Here's how the part is built. I have some questions about the finished solid (model axes, mm). A direction names the side the tool comes from. Round coordinates to 2 decimals unless told otherwise and drop trailing zeros. Order: outer loops, then holes, each group sorted by start corner. A loop starts at its lowest first (then second) coordinate and runs counter-clockwise, first axis right, second up. Notation, with made-up numbers: M 30,31.25 L 62,31.25 A20 cw 62,42.25 Z; hole C 63.5,32.25 d1. An arc over 180 degrees is marked long. Write item = value, one per line. Start each with the question number.
Item 1: For faces 4 (the face through (-0.43, 61.27, 6.06)), 5 (the face through (-13, 10, -21)), 6 (the face through (13.3, 0.1, 21.8)), which set-ups out of +Z, -Z, +X, -X, +Y, -Y let a thin tool reach every point of the face, with its end or its side?
Item 2: I want a section at D-D, the plane x = 0. State how many separate pieces and enclosed holes the cut face has, plus the area to 3 significant figures.
Item 3: We'd pull the mould along Z, two halves only. Please class faces 1 (the face through (-13, 0, 26)), 2 (the face through (-0.254, 31.933, -3.916)), 3 (the face through (0.228, 49.266, -1.292)): pulls with the +Z half, pulls with the -Z half, needs draft (parallel to the pull), parting line crosses it, or undercut.
Item 4: I'm going to push flat-ended pins straight in: P1, Ø3, axis at x = -9, y = 24.5, coming from the +Z side; P2, Ø5, axis at y = 0, z = -19, coming from the +X side; P3, Ø1.8, axis at x = 13.5, z = 20.5, coming from the +Y side; P4, Ø10, axis at x = -3, z = 2, coming from the -Y side. Where does each tip first touch, or does it pass through?
Item 5: Please list where these lines run through material, in increasing order: L1, parallel to Y at x = 0, z = -7.25; L2, parallel to Y at x = 9, z = 0; L3, parallel to Y at x = -3, z = -1.5.
Item 6: I want a section at A-A, the plane x = -9. List the corners of the cut face in (y, z) for me.
Item 7: I want a section at B-B, the plane y = 58. List the corners of the cut face in (x, z) for me.
Item 8: I want a section at C-C, the plane z = 19. List the corners of the cut face in (x, y) for me.
```python
from build123d import *

# Parameters (mm, degrees)
EXTRUDE1_DEPTH      = 10.3
EXTRUDE1_DEPTH_BACK = 10.3
SKETCH1_W           = 20
SKETCH1_H           = 55
EXTRUDE2_DEPTH      = 6
SKETCH4_R           = 2.8
EXTRUDE3_DEPTH      = 78.478061411
SKETCH5_R           = 5
EXTRUDE4_DEPTH      = 77.326797391
FILLET2_R           = 1.5
CHAMFER1_SIZE       = 2
SKETCH7_R           = 1.95
EXTRUDE5_DEPTH      = 77.326797413
SKETCH8_R           = 3.3
EXTRUDE6_DEPTH      = 8


with BuildPart() as part:
    # Sketch1 → Extrude1 (new, two sides: drawn at the far end of the back side and taken through both)
    with BuildSketch(Plane(origin=(0, 0, 0), x_dir=(0, 0, -1), z_dir=(1, 0, 0)).offset(-EXTRUDE1_DEPTH_BACK)):
        with Locations((0, 37.8)):
            Rectangle(SKETCH1_W, SKETCH1_H)
    extrude(amount=EXTRUDE1_DEPTH + EXTRUDE1_DEPTH_BACK)

    # Sketch2 → Extrude2 (add)
    with BuildSketch(Plane(origin=(10.3, 0, 0), x_dir=(0, 0, -1), z_dir=(1, 0, 0))):
        with BuildLine():
            Line((26, 10), (17, 10))
            ThreePointArc((17, 10), (12.050252532, 12.050252532), (10, 17))
            Line((10, 17), (10, 65.3))
            Line((10, 65.3), (-10, 65.3))
            Line((-10, 65.3), (-10, 17))
            ThreePointArc((-10, 17), (-12.050252532, 12.050252532), (-17, 10))
            Line((-17, 10), (-26, 10))
            Line((-26, 10), (-26, -10))
            Line((-26, -10), (26, -10))
            Line((26, -10), (26, 10))
        make_face()
    extrude2 = extrude(amount=EXTRUDE2_DEPTH)

    # Mirror2: Extrude2 across plane
    add(extrude2.mirror(Plane(origin=(0, 0, 0), x_dir=(0, 0, 1), z_dir=(1, 0, 0))))

    # Sketch4 → Extrude3 (cut, through all)
    with BuildSketch(Plane(origin=(16.3, 0, 0), x_dir=(0, 0, -1), z_dir=(1, 0, 0))):
        Circle(SKETCH4_R)
        with Locations((19, 0)):
            Circle(SKETCH4_R)
        with Locations((-19, 0)):
            Circle(SKETCH4_R)
        with Locations((0, 19.5)):
            Circle(SKETCH4_R)
        with Locations((0, 51.75)):
            Circle(SKETCH4_R)
    extrude(amount=-EXTRUDE3_DEPTH, mode=Mode.SUBTRACT)

    # Sketch5 → Extrude4 (cut, through all)
    with BuildSketch(Plane.XY.offset(10)):
        with Locations((0, 44)):
            Circle(SKETCH5_R)
    extrude(amount=-EXTRUDE4_DEPTH, mode=Mode.SUBTRACT)

    # Fillet2
    fillet2_edges = [part.edges().sort_by_distance(p)[0] for p in [
        (13.3, 10, 26),
        (13.3, -10, 26),
        (13.3, -10, -26),
        (13.3, 10, -26),
        (-13.3, -10, 26),
        (-13.3, 10, 26),
        (-13.3, 10, -26),
        (-13.3, -10, -26),
        (0, 65.3, 10),
        (0, 65.3, -10),
    ]]
    fillet(fillet2_edges, radius=FILLET2_R)

    # Chamfer1
    chamfer1_edges = [part.edges().sort_by_distance(p)[0] for p in [
        (-5, 44, -10),
        (-5, 44, 10),
    ]]
    chamfer(chamfer1_edges, length=CHAMFER1_SIZE)

    # Sketch7 → Extrude5 (cut, through all)
    with BuildSketch(Plane.XY.offset(10)):
        with Locations((0, 58)):
            Circle(SKETCH7_R)
        with Locations((0, 30)):
            Circle(SKETCH7_R)
    extrude(amount=-EXTRUDE5_DEPTH, mode=Mode.SUBTRACT)

    # Sketch8 → Extrude6 (cut)
    with BuildSketch(Plane.XY.offset(10)):
        with Locations((0, 58)):
            Circle(SKETCH8_R)
        with Locations((0, 30)):
            Circle(SKETCH8_R)
    extrude(amount=-EXTRUDE6_DEPTH, mode=Mode.SUBTRACT)


solid = part.part
```
Filled in:
q1.face_4 = +Z
q1.face_5 = -Z, +X, -X, +Y
q1.face_6 = +X, -X
q2.separate_pieces = 4
q2.enclosed_holes = 1
q2.area = 643 mm^2
q3.face_1 = pulls with the +Z half
q3.face_2 = needs draft
q3.face_3 = undercut
q4.P1 = 10
q4.P2 = through
q4.P3 = 10
q4.P4 = 10.3
q5.L1 = 10.3 to 28.05, 31.95 to 39, 49 to 56.05, 59.95 to 65.3
q5.L2 = 10.3 to 16.7, 22.3 to 48.95, 54.55 to 65.3
q5.L3 = 10.3 to 17.14, 21.86 to 40, 48 to 49.39, 54.11 to 65.3
q6.outline = M 10.3,-10 L 63.8,-10 A1.5 ccw 65.3,-8.5 L 65.3,8.5 A1.5 ccw 63.8,10 L 10.3,10 Z; hole C 19.5,0 d5.6; hole C 51.75,0 d5.6
q7.outline = M -16.3,-10 L -1.95,-10 L -1.95,2 L -3.3,2 L -3.3,10 L -16.3,10 Z; M 1.95,-10 L 16.3,-10 L 16.3,10 L 3.3,10 L 3.3,2 L 1.95,2 Z
q8.outline = M -16.3,-10 L -10.3,-10 L -10.3,-2.8 L -16.3,-2.8 Z; M -16.3,2.8 L -10.3,2.8 L -10.3,10 L -16.3,10 Z; M 10.3,-10 L 16.3,-10 L 16.3,-2.8 L 10.3,-2.8 Z; M 10.3,2.8 L 16.3,2.8 L 16.3,10 L 10.3,10 Z
